Autodesk Fusion 360 part; units mm, degrees
sketch "Sketch1" plane through (0, 0, 0) normal (0, 0, 1) x (1, 0, 0)
  line L0 (-2, 1.8875) -> (-2, -1.8875)
  line L1 (2, -1.8875) -> (2, 1.8875)
  line L2 (1.0213, 2.5533) -> (-1.0213, -2.5533) construction
  line L3 (-1.0213, 2.5533) -> (1.0213, -2.5533) construction
  arc A0 (2, 1.8875) -> (-2, 1.8875) centre (0, 0) ccw
  arc A1 (-2, -1.8875) -> (2, -1.8875) centre (0, 0) ccw
  circle A2 centre (0, 0) radius 6
  dimension "d1" = 5.5
  dimension "d4" = 12
extrude "Extrude1" add sketch "Sketch1" along normal blind 7
chamfer "Chamfer1" distance 2 angle 45 1 edges at (-5.594, -2.1697, 0)
sketch "Sketch2" plane through (0, 0, 7) normal (0, 0, 1) x (-1, 0, 0)
  arc A0 (2, 1.8875) -> (-2, 1.8875) centre (0, 0) ccw
  line L0 (2, 1.8875) -> (2, -1.8875)
  arc A1 (-2, -1.8875) -> (2, -1.8875) centre (0, 0) ccw
  line L1 (-2, -1.8875) -> (-2, 1.8875)
  circle A2 centre (0, 0) radius 6
  circle A3 centre (0, 0) radius 7.5
  dimension "d8" = 15
extrude "Extrude2" add sketch "Sketch2" along normal blind 6 contours A2 | A3
sketch "Sketch3" plane through (0, 0, 13) normal (0, 0, 1) x (-1, 0, 0)
  arc A0 (2, 1.8875) -> (-2, 1.8875) centre (0, 0) ccw
  line L0 (2, 1.8875) -> (2, -1.8875)
  arc A1 (-2, -1.8875) -> (2, -1.8875) centre (0, 0) ccw
  line L1 (-2, -1.8875) -> (-2, 1.8875)
  circle A2 centre (0, 0) radius 7.5
  line L2 (0, -7.5) -> (0, -17.5) construction
  line L3 (0, -17.5) -> (5, -17.5) construction
  line L4 (5, -17.5) -> (-5, -17.5) construction
  line L5 (-5, -17.5) -> (-5, -5.5902) construction
  line L6 (5, -17.5) -> (5, -5.5902) construction
  line L7 (5, -5.5902) -> (5, -17.5)
  line L8 (-5, -17.5) -> (-5, -5.5902)
  line L9 (-5, -17.5) -> (5, -17.5)
  line L10 (17.6554, 4.4199) -> (7.3412, -1.535)
  line L11 (17.6554, 4.4199) -> (12.6554, 13.0801)
  line L12 (12.6554, 13.0801) -> (2.3412, 7.1252) construction
  line L13 (-12.6554, 13.0801) -> (-2.3412, 7.1252)
  line L14 (-12.6554, 13.0801) -> (-17.6554, 4.4199)
  line L15 (-17.6554, 4.4199) -> (-7.3412, -1.535) construction
  line L16 (-7.3412, -1.535) -> (-17.6554, 4.4199)
  line L17 (2.3412, 7.1252) -> (12.6554, 13.0801)
  dimension "d11" = 10
  dimension "d12" = 5
  dimension "d18" = 360
extrude "Extrude3" add sketch "Sketch3" against normal blind 6 contours A2 L7 L8 L9
fillet "Fillet1" radius 5 2 edges at (5, 17.5, 10) (-5, 17.5, 10)
extrude "Extrude4" add sketch "Sketch3" against normal blind 6 contours A2 L10 L11 L17 | A2 L13 L14 L16 | A2 L7 L8 L9
fillet "Fillet2" radius 4 6 edges at (-5, 17.5, 10) (5, 17.5, 10) (17.6554, -4.4199, 10) (12.6554, -13.0801, 10) (-12.6554, -13.0801, 10) (-17.6554, -4.4199, 10)
sketch "Sketch4" plane through (0, 0, 13) normal (0, 0, 1) x (-1, 0, 0)
  arc A0 (14.1913, 2.4199) -> (15.6554, 7.884) centre (12.1913, 5.884) ccw
  line L0 (15.6554, 7.884) -> (14.6554, 9.616)
  arc A1 (14.6554, 9.616) -> (9.1913, 11.0801) centre (11.1913, 7.616) ccw
  line L1 (9.1913, 11.0801) -> (2.3412, 7.1252)
  arc A2 (2.3412, 7.1252) -> (-2.3412, 7.1252) centre (0, 0) ccw
  line L2 (-2.3412, 7.1252) -> (-9.1913, 11.0801)
  arc A3 (-9.1913, 11.0801) -> (-14.6554, 9.616) centre (-11.1913, 7.616) ccw
  line L3 (-14.6554, 9.616) -> (-15.6554, 7.884)
  arc A4 (-15.6554, 7.884) -> (-14.1913, 2.4199) centre (-12.1913, 5.884) ccw
  line L4 (-14.1913, 2.4199) -> (-7.3412, -1.535)
  arc A5 (-7.3412, -1.535) -> (-5, -5.5902) centre (0, 0) ccw
  line L5 (-5, -5.5902) -> (-5, -13.5)
  arc A6 (-5, -13.5) -> (-1, -17.5) centre (-1, -13.5) ccw
  line L6 (-1, -17.5) -> (1, -17.5)
  arc A7 (1, -17.5) -> (5, -13.5) centre (1, -13.5) ccw
  line L7 (5, -13.5) -> (5, -5.5902)
  arc A8 (5, -5.5902) -> (7.3412, -1.535) centre (0, 0) ccw
  line L8 (7.3412, -1.535) -> (14.1913, 2.4199)
  arc A9 (2, 1.8875) -> (-2, 1.8875) centre (0, 0) ccw
  line L9 (2, 1.8875) -> (2, -1.8875)
  arc A10 (-2, -1.8875) -> (2, -1.8875) centre (0, 0) ccw
  line L10 (-2, -1.8875) -> (-2, 1.8875)
  circle A11 centre (0, 0) radius 20
  dimension "d23" = 40
extrude "Extrude5" add sketch "Sketch4" along normal blind 4 contours A0 L0 A1 L1 A2 L2 A3 L3 A4 L4 A5 L5 A6 L6 A7 L7 A8 L8 | A9 L9 A10 L10 | A11
chamfer "Chamfer2" distance 2 angle 45 1 edges at (18.6465, 7.2323, 17)
sketch "Sketch5" plane through (0, 0, 7) normal (0, 0, -1) x (1, 0, 0)
  arc A0 (-15.6554, 7.884) -> (-14.1913, 2.4199) centre (-12.1913, 5.884) ccw
  line L0 (-14.1913, 2.4199) -> (-7.3412, -1.535)
  arc A1 (-7.3412, -1.535) -> (-5, -5.5902) centre (0, 0) ccw
  line L1 (-5, -5.5902) -> (-5, -13.5)
  arc A2 (-5, -13.5) -> (-1, -17.5) centre (-1, -13.5) ccw
  line L2 (-1, -17.5) -> (1, -17.5)
  arc A3 (1, -17.5) -> (5, -13.5) centre (1, -13.5) ccw
  line L3 (5, -13.5) -> (5, -5.5902)
  arc A4 (5, -5.5902) -> (7.3412, -1.535) centre (0, 0) ccw
  line L4 (7.3412, -1.535) -> (14.1913, 2.4199)
  arc A5 (14.1913, 2.4199) -> (15.6554, 7.884) centre (12.1913, 5.884) ccw
  line L5 (15.6554, 7.884) -> (14.6554, 9.616)
  arc A6 (14.6554, 9.616) -> (9.1913, 11.0801) centre (11.1913, 7.616) ccw
  line L6 (9.1913, 11.0801) -> (2.3412, 7.1252)
  arc A7 (2.3412, 7.1252) -> (-2.3412, 7.1252) centre (0, 0) ccw
  line L7 (-2.3412, 7.1252) -> (-9.1913, 11.0801)
  arc A8 (-9.1913, 11.0801) -> (-14.6554, 9.616) centre (-11.1913, 7.616) ccw
  line L8 (-14.6554, 9.616) -> (-15.6554, 7.884)
  circle A9 centre (0, 0) radius 6
Read the model definition and answer for the solid it produces. Units are mm, in the model's axes. A direction names the side the tool comes from. Round coordinates to 2 decimals unless told otherwise and drop trailing zeros. Write each loop counter-clockwise with the first axis right and the second up, starting at its lowest first coordinate (ties: lowest second). Pieces come first, ordered by that corner, then holes. Notation, with made-up numbers: M 27.25,-2.75 L 79.25,-2.75 A19 ccw 79.25,2.25 Z; hole C -37,38 d6. An arc over 180 degrees is marked long. Use a Markdown table: item, result.
1) The part is cut by section D-D (y = 0). Write down the section's boundary in (x, z).
Answers follow:
| item | result |
|---|---|
| outline | M -20,13 L -10,13 L -10,7 L -6,7 L -6,2 L -4,0 L -2,0 L -2,13 L 2,13 L 2,0 L 4,0 L 6,2 L 6,7 L 10,7 L 10,13 L 20,13 L 20,15 L 18,17 L -18,17 L -20,15 Z |
2) The part is cut by section A-A (z = 1.25). Write down the section's boundary in (x, y).
Answers follow:
| item | result |
|---|---|
| outline | C 0,0 d10.5; hole M -2,-1.89 A2.75 ccw 2,-1.89 L 2,1.89 A2.75 ccw -2,1.89 Z |
3) The part is cut by section C-C (z = 5.75). Write down the section's boundary in (x, y), plus the area to 3 significant figures.
Answers follow:
| item | result |
|---|---|
| outline | C 0,0 d12; hole M -2,-1.89 A2.75 ccw 2,-1.89 L 2,1.89 A2.75 ccw -2,1.89 Z |
| area | 93.2 mm2 |
4) For a pull along Y with two mould halves and no side action, classify faces 5 (the flat face through (10.718, -0.415, 10.042)), 6 (the cylindrical face through (-6, 0, 4)), 7 (the flat face through (0, 0, 13)), 8 (the flat face through (-5, 9, 10)) as pulls with the +Y half, pulls with the -Y half, needs draft (parallel to the pull), parting line crosses it, or undercut.
Answers follow:
| item | result |
|---|---|
| face 5 | pulls with the +Y half |
| face 6 | parting line crosses it |
| face 7 | undercut |
| face 8 | needs draft |
5) A tool of negligible diameter and unlimited length cuts with its end or side. For faces 1 (the flat face through (15.15, -8.76, 10.04)), 2 (the cylindrical face through (0, -7.5, 10)), 3 (the cylindrical face through (3.797, 16.359, 9.958)), 4 (the flat face through (2, 0, 6)), from which of +Z, -Z, +X, -X, +Y, -Y can it reach the whole face along a straight path? Write none if from no direction.
Answers follow:
| item | result |
|---|---|
| face 1 | -Z, +X, -Y |
| face 2 | -Z, -Y |
| face 3 | -Z, +X, +Y |
| face 4 | -Z |
6) Straight lines are drawn through the part: line 1 along Z through (x, y) = (-11.5, -13); line 2 along X through (y, z) = (2.5, 6.5); line 3 along X through (y, z) = (8, 10.75). For each, find the intervals that lie inside material, in ascending order. Write a range as [from, to].
Answers follow:
| item | result |
|---|---|
| line 1 | z = [13, 17] |
| line 2 | x = [-5.45, -1.15], [1.15, 5.45] |
| line 3 | x = [-5, 5] |
7) The part is cut by section B-B (x = 0). Write down the section's boundary in (y, z).
Answers follow:
| item | result |
|---|---|
| outline | M -20,13 L -7.5,13 L -7.5,7 L -6,7 L -6,2 L -4,0 L -2.75,0 L -2.75,13 L 2.75,13 L 2.75,0 L 4,0 L 6,2 L 6,7 L 17.5,7 L 17.5,13 L 20,13 L 20,15 L 18,17 L -18,17 L -20,15 Z |
8) Flat-ended cylindrical pins translate along their axes: pin 1 (8 mm diameter, centred on x = 15.5, z = 8, fed in from -Y); pin 2 (23.5 mm diameter, centred on x = 2, y = 6, fed in from -Z); pin 3 (1.8 mm diameter, centred on y = 8.5, z = 10.5, fed in from -X); pin 4 (1.9 mm diameter, centred on y = 0, z = 4.5, fed in from +X). Find the tip coordinate at first contact, or state that the pin passes through.
Answers follow:
| item | result |
|---|---|
| pin 1 | stops at y = -11.6 |
| pin 2 | stops at z = 0 |
| pin 3 | stops at x = -5 |
| pin 4 | stops at x = 6 |
